from build123d import *

# Parameters (mm, degrees)
SKETCH1_W           = 30
SKETCH1_H           = 30
SKETCH1_W_2         = 26
SKETCH1_H_2         = 26
BOSS_EXTRUDE1_DEPTH = 300
SKETCH2_R           = 12
SKETCH2_R_2         = 10
BOSS_EXTRUDE2_DEPTH = 5
SKETCH3_R           = 12
SKETCH3_R_2         = 10
BOSS_EXTRUDE3_DEPTH = 5


with BuildPart() as part:
    # Sketch1 → Boss-Extrude1 (new body)
    with BuildSketch(Plane.XY):
        Rectangle(SKETCH1_W, SKETCH1_H)
        Rectangle(SKETCH1_W_2, SKETCH1_H_2, mode=Mode.SUBTRACT)
    extrude(amount=BOSS_EXTRUDE1_DEPTH)

    # Sketch2 → Boss-Extrude2 (add)
    with BuildSketch(Plane(origin=(15, 0, 0), x_dir=(0, 0, -1), z_dir=(1, 0, 0))):
        with Locations(Location((-15, 0, 0), (0, 0, 180))):
            Circle(SKETCH2_R)
        with Locations((-15, 0)):
            Circle(SKETCH2_R_2, mode=Mode.SUBTRACT)
    extrude(amount=BOSS_EXTRUDE2_DEPTH)

    # Sketch3 → Boss-Extrude3 (add)
    with BuildSketch(Plane.ZY.offset(15)):
        with Locations(Location((275, 0, 0), (0, 0, 180))):
            Circle(SKETCH3_R)
        with Locations((275, 0)):
            Circle(SKETCH3_R_2, mode=Mode.SUBTRACT)
    extrude(amount=BOSS_EXTRUDE3_DEPTH)


solid = part.part
Model file for the job. Use its own axes, mm. A direction names the side the tool comes from. Round coordinates to 2 decimals unless told otherwise and drop trailing zeros. Loops run counter-clockwise (first coordinate to the right, second up) from the corner with the lowest first, then second, coordinate; pieces in that order, holes last. Notation, with made-up numbers: (-8, -5.5) - (11, -5.5) arc R15 cw to (11, 14.5) - close; hole circle Ø10 at (24.5, 82.5). An arc over 180 degrees is marked (long way). Write each question's results on one line, items separated by ' | '.
(1) Mould opens along Y. For faces 5 (the flat face through (15, 0, 148)), 6 (the flat face through (0, -15, 148)), 7 (the flat face through (0, -13, 148)) say: released by +Y, released by -Y, zero draft, split by the parting line, or undercut.
Answer below:
face 5: zero draft | face 6: released by -Y | face 7: undercut
(2) Saw through at B-B, the plane x = 0.5. List the corners of the cut face in (y, z).
Answer below:
outline: (-15, 0) - (-13, 0) - (-13, 300) - (-15, 300) - close; (13, 0) - (15, 0) - (15, 300) - (13, 300) - close
(3) Saw through at D-D, the plane z = 15. List the corners of the cut face in (x, y), then the cut area to 3 significant figures.
Answer below:
outline: (-15, -15) - (15, -15) - (15, -12) - (20, -12) - (20, -10) - (15, -10) - (15, 10) - (20, 10) - (20, 12) - (15, 12) - (15, 15) - (-15, 15) - close; hole (-13, -13) - (13, -13) - (13, 13) - (-13, 13) - close | area: 244 mm^2
(4) Saw through at A-A, the plane z = 96.5. List the corners of the cut face in (x, y).
Answer below:
outline: (-15, -15) - (15, -15) - (15, 15) - (-15, 15) - close; hole (-13, -13) - (13, -13) - (13, 13) - (-13, 13) - close
(5) Wall check: L1, parallel to X at y = 8.25, z = 279; L2, parallel to Y at x = 18, z = 15. Give the ranges that are in metal, low to high.
Answer below:
L1: x = -15 to -13, 13 to 15 | L2: y = -12 to -10, 10 to 12
(6) Pin check, flat tips, straight feed: pin 1 (8 mm diameter, centred on y = -3.5, z = 128.5, fed in from +X); pin 2 (4 mm diameter, centred on y = 2, z = 41, fed in from -X); pin 3 (1.5 mm diameter, centred on x = -16, z = 235, fed in from +Y). Stop position of each tip, or through.
Answer below:
pin 1: stops at x = 15 | pin 2: stops at x = -15 | pin 3: passes through
(7) 3-axis set-ups, long thin cutter, end or side, ignore diameter. For faces 1 (the cylindrical face through (-17.465, 7.302, 284.523)), 2 (the flat face through (-14, 0, 0)), 3 (the cylindrical face through (17.46, 3, 5.46)), 4 (the flat face through (-13, 0, 148)): which of +Z, -Z, +X, -X, +Y, -Y reach the whole face in a straight line?
Answer below:
face 1: -X | face 2: -Z, +X, -X, +Y, -Y | face 3: +X | face 4: +Z, -Z
(8) Saw through at C-C, the plane y = 0. List the corners of the cut face in (x, z).
Answer below:
outline: (-20, 263) - (-15, 263) - (-15, 0) - (-13, 0) - (-13, 300) - (-15, 300) - (-15, 287) - (-20, 287) - (-20, 285) - (-15, 285) - (-15, 265) - (-20, 265) - close; (13, 0) - (15, 0) - (15, 3) - (20, 3) - (20, 5) - (15, 5) - (15, 25) - (20, 25) - (20, 27) - (15, 27) - (15, 300) - (13, 300) - close
